The listing builds one solid part. Answer for the finished solid, in the listing's coordinates (mm). A direction names the side the tool comes from. Give positions to 0.01 mm unless a question says otherwise; leave off trailing zeros. Loops run counter-clockwise (first coordinate to the right, second up) from the corner with the lowest first, then second, coordinate; pieces in that order, holes last. Notation, with made-up numbers: (10, 52) - (40, 52) arc R13 cw to (40, 57) - close; hole circle Ø3 at (79, 11.5). An arc over 180 degrees is marked (long way). Write item = value, one per line. Start each with the question number.
1) The part is cut by section B-B on x = 95. Write down the section's boundary in (y, z).
2) The part is cut by section D-D on x = 14.5. Write down the section's boundary in (y, z).
3) The part is cut by section A-A on y = 5. Write down the section's boundary in (x, z), plus the area to 3 significant figures.
4) Which of the six approach directions +Z, -Z, +X, -X, +Y, -Y give full straight-line access (tool end or side, diameter ignored) to faces 1 (the flat face through (50, 30, -6)), 2 (the flat face through (50, 20, -6)), 3 (the cylindrical face through (4.46, 42.56, -0.07)), 4 (the flat face through (60, 25, -6))?
5) The mould has two halves that part along X. Classify faces 5 (the cylindrical face through (92.5, 5.1, -0.1)), 6 (the cylindrical face through (93, 43.5, -0.1)), 7 (the flat face through (40, 25, -6)), 8 (the flat face through (49, 25, 5)): +X half, -X half, draft (parallel to the pull), parting line (faces both ways), or undercut.
6) The part is cut by section C-C on z = 3.5. Write down the section's boundary in (x, y).
7) Consider probe 1 along Y at (x, z) = (5, -2.25); probe 2 along X at (y, z) = (43.5, 0); probe 3 along X at (y, z) = (7, 0.75). Determine where each line is inside the solid, lowest interval first.
8) Flat-ended cylindrical pins translate along their axes: P1, Ø1.1, axis at x = 53.5, z = -7.5, coming from the -Y side; P2, Ø3, axis at x = 5, y = 5, coming from the -Z side; P3, Ø5, axis at x = 18.5, z = 1, coming from the -Y side; P4, Ø0.5, axis at y = 25, z = -7.5, coming from the +X side. Find the tip coordinate at first contact, or state that the pin passes through.
from build123d import *

# Parameters (mm, degrees)
SKETCH1_W           = 100
SKETCH1_H           = 50
SKETCH1_R           = 2.5
BOSS_EXTRUDE1_DEPTH = 5
SKETCH2_W           = 20
SKETCH2_H           = 10
SKETCH2_W_2         = 8.5
SKETCH2_H_2         = 8
BOSS_EXTRUDE2_DEPTH = 2
SKETCH2_3_W         = 8.5
SKETCH2_3_H         = 8
BOSS_EXTRUDE3_DEPTH = 3


with BuildPart() as part:
    # Sketch1 → Boss-Extrude1 (new, symmetric)
    with BuildSketch(Plane.XY):
        with Locations((50, 25)):
            Rectangle(SKETCH1_W, SKETCH1_H)
        with Locations((5, 5)):
            Circle(SKETCH1_R, mode=Mode.SUBTRACT)
        with Locations((5, 45)):
            Circle(SKETCH1_R, mode=Mode.SUBTRACT)
        with Locations((95, 45)):
            Circle(SKETCH1_R, mode=Mode.SUBTRACT)
        with Locations((95, 5)):
            Circle(SKETCH1_R, mode=Mode.SUBTRACT)
    extrude(amount=BOSS_EXTRUDE1_DEPTH, both=True)

    # Sketch2 → Boss-Extrude2 (add)
    with BuildSketch(Plane(origin=(0, 0, -5), x_dir=(-1, 0, 0), z_dir=(0, 0, -1))):
        with Locations((-50, 25)):
            Rectangle(SKETCH2_W, SKETCH2_H)
        with Locations((-54.75, 25)):
            Rectangle(SKETCH2_W_2, SKETCH2_H_2, mode=Mode.SUBTRACT)
        with Locations((-45.25, 25)):
            Rectangle(SKETCH2_W_2, SKETCH2_H_2, mode=Mode.SUBTRACT)
    extrude(amount=BOSS_EXTRUDE2_DEPTH)

    # Sketch2<3> → Boss-Extrude3 (add)
    with BuildSketch(Plane(origin=(0, 0, -5), x_dir=(-1, 0, 0), z_dir=(0, 0, -1))):
        with Locations((-54.75, 25)):
            Rectangle(SKETCH2_3_W, SKETCH2_3_H)
        with Locations((-45.25, 25)):
            Rectangle(SKETCH2_3_W, SKETCH2_3_H)
    extrude(amount=BOSS_EXTRUDE3_DEPTH)


solid = part.part
Answer below:
q1.outline = (0, -5) - (2.5, -5) - (2.5, 5) - (0, 5) - close; (7.5, -5) - (42.5, -5) - (42.5, 5) - (7.5, 5) - close; (47.5, -5) - (50, -5) - (50, 5) - (47.5, 5) - close
q2.outline = (0, -5) - (50, -5) - (50, 5) - (0, 5) - close
q3.outline = (0, -5) - (2.5, -5) - (2.5, 5) - (0, 5) - close; (7.5, -5) - (92.5, -5) - (92.5, 5) - (7.5, 5) - close; (97.5, -5) - (100, -5) - (100, 5) - (97.5, 5) - close
q3.area = 900 mm2
q4.face_1 = -Z, +X, -X, +Y
q4.face_2 = -Z, +X, -X, -Y
q4.face_3 = +Z, -Z
q4.face_4 = -Z, +X, +Y, -Y
q5.face_5 = undercut
q5.face_6 = undercut
q5.face_7 = -X half
q5.face_8 = draft
q6.outline = (0, 0) - (100, 0) - (100, 50) - (0, 50) - close; hole circle Ø5 at (5, 5); hole circle Ø5 at (5, 45); hole circle Ø5 at (95, 5); hole circle Ø5 at (95, 45)
q7.probe_1 = 0 to 2.5, 7.5 to 42.5, 47.5 to 50
q7.probe_2 = 0 to 3, 7 to 93, 97 to 100
q7.probe_3 = 0 to 3.5, 6.5 to 93.5, 96.5 to 100
q8.P1 = 20
q8.P2 = through
q8.P3 = 0
q8.P4 = 59
